Geometry check sheet. Reference: drawing and pictorial views, mm from the part's lowest x, y, z. Round coordinates to 2 decimals unless told otherwise and drop trailing zeros. Loops run counter-clockwise (first coordinate to the right, second up) from the corner with the lowest first, then second, coordinate; pieces in that order, holes last. Notation, with made-up numbers: (78, 12) -> (106, 12) arc R21 ccw to (106, 45) -> close; hole circle Ø4 at (78.25, -18.5). An arc over 180 degrees is marked (long way). Use one line per item in the form item = value. Start each with the question number.
(1) Go/stop test with flat-tipped pins: pin 1 (10 mm diameter, centred on y = 99.5, z = 21, fed in from -X); pin 2 (1 mm diameter, centred on x = 51.5, z = 13, fed in from +Y); pin 3 (5 mm diameter, centred on y = 105.5, z = 19, fed in from -X) (1 decimal). Record where each tip stops, or that it passes through.
(2) Sectioned sample at D-D (z = 26.5). Record the cut outline in (x, y), and give its area (3 significant figures).
(3) Draft check along Y on the marked faces 1, 2 and 3. Enter one of: released by +Y, released by -Y, zero draft, split by the parting line, or undercut.
(4) Material ranges on probe 1 along Y at (x, z) = (59, 18); probe 2 along Y at (x, z) = (59, 28) (1 decimal); probe 3 along X at (y, z) = (48.5, 31.5) (1 decimal), recorded low to high. Write a range as [from, to].
(5) Sectioned sample at C-C (z = 15). Record the cut outline in (x, y), and give its area (3 significant figures).
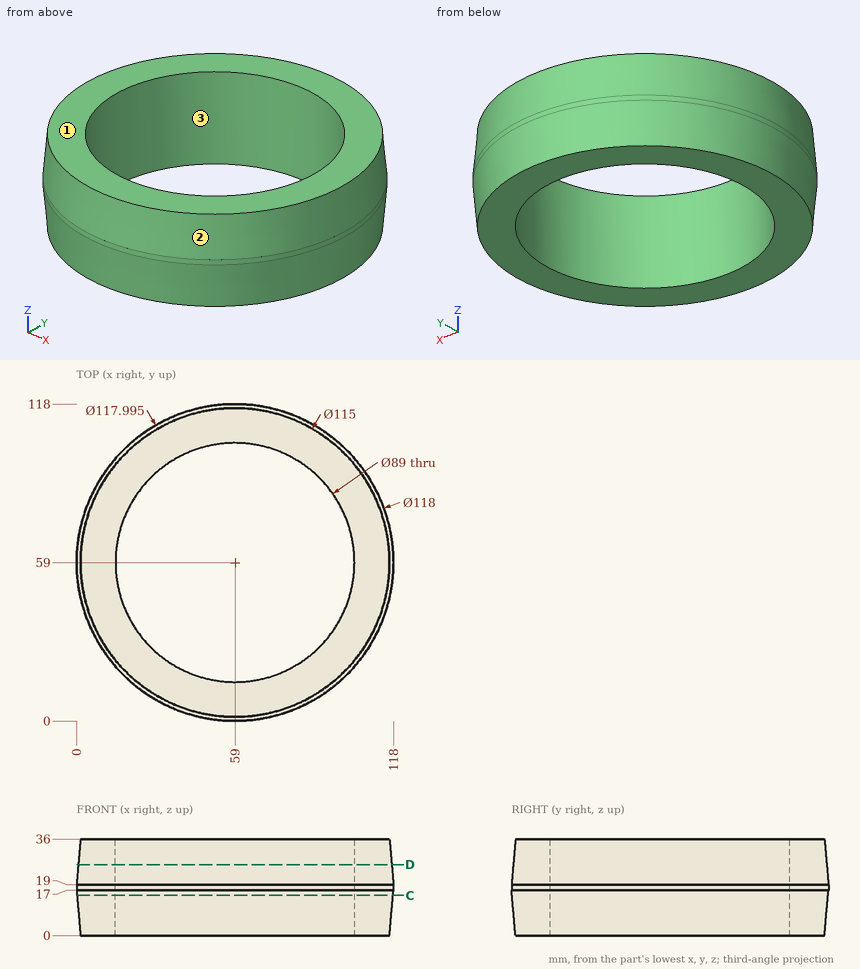
Checks:
q1.pin_1 = 12.06
q1.pin_2 = 117.24
q1.pin_3 = 19.7
q2.outline = circle Ø116.67 at (59, 59); hole circle Ø89 at (59, 59)
q2.area = 4,470 mm2
q3.face_1 = zero draft
q3.face_2 = split by the parting line
q3.face_3 = undercut
q4.probe_1 = [0, 14.5], [103.5, 118]
q4.probe_2 = [0.8, 14.5], [103.5, 117.2]
q4.probe_3 = [2.1, 15.8], [102.2, 115.9]
q5.outline = circle Ø117.65 at (59, 59); hole circle Ø89 at (59, 59)
q5.area = 4,650 mm2
